from build123d import *

# Parameters (mm, degrees)
BOSS_EXTRUDE1_DEPTH   = 3
CUT_EXTRUDE1_REACH    = 84.517
SKETCH2_R             = 1
SKETCH2_R_2           = 1.25
SKETCH3_R             = 10
BOSS_EXTRUDE2_DEPTH   = 15
BODY_MOVE_COPY2_ANGLE = 90


with BuildPart() as part:
    # Sketch1 → Boss-Extrude1 (new body)
    with BuildSketch(Plane(origin=(0, 0, 0), x_dir=(1, 0, 0), z_dir=(0, 1, 0))):
        with BuildLine():
            Line((60, -20), (0, -20))
            ThreePointArc((0, -20), (-20, 0), (0, 20))
            Line((0, 20), (60, 20))
            Line((60, 20), (80, 0))
            Line((80, 0), (60, -20))
        make_face()
    extrude(amount=BOSS_EXTRUDE1_DEPTH)

    # Sketch2 → Cut-Extrude1 (cut, up to next)
    with BuildSketch(Plane(origin=(0, 3, 0), x_dir=(1, 0, 0), z_dir=(0, 1, 0)), mode=Mode.PRIVATE) as cut_extrude1_sk1:
        with Locations(Location((0, 0, 0), (0, 0, 270))):
            Circle(SKETCH2_R)
    cut_extrude1_tool1 = extrude(cut_extrude1_sk1.sketch, amount=-CUT_EXTRUDE1_REACH, mode=Mode.PRIVATE) & part.part
    # Sketch2 → Cut-Extrude1 (cut, up to next)
    with BuildSketch(Plane(origin=(0, 3, 0), x_dir=(1, 0, 0), z_dir=(0, 1, 0)), mode=Mode.PRIVATE) as cut_extrude1_sk2:
        with Locations(Location((0, 7, 0), (0, 0, 270))):
            Circle(SKETCH2_R_2)
    cut_extrude1_tool2 = extrude(cut_extrude1_sk2.sketch, amount=-CUT_EXTRUDE1_REACH, mode=Mode.PRIVATE) & part.part
    # Sketch2 → Cut-Extrude1 (cut, up to next)
    with BuildSketch(Plane(origin=(0, 3, 0), x_dir=(1, 0, 0), z_dir=(0, 1, 0)), mode=Mode.PRIVATE) as cut_extrude1_sk3:
        with Locations(Location((7.001, 0.001, 0), (0, 0, 270))):
            Circle(SKETCH2_R_2)
    cut_extrude1_tool3 = extrude(cut_extrude1_sk3.sketch, amount=-CUT_EXTRUDE1_REACH, mode=Mode.PRIVATE) & part.part
    # Sketch2 → Cut-Extrude1 (cut, up to next)
    with BuildSketch(Plane(origin=(0, 3, 0), x_dir=(1, 0, 0), z_dir=(0, 1, 0)), mode=Mode.PRIVATE) as cut_extrude1_sk4:
        with Locations(Location((0.002, -7, 0), (0, 0, 270))):
            Circle(SKETCH2_R_2)
    cut_extrude1_tool4 = extrude(cut_extrude1_sk4.sketch, amount=-CUT_EXTRUDE1_REACH, mode=Mode.PRIVATE) & part.part
    # Sketch2 → Cut-Extrude1 (cut, up to next)
    with BuildSketch(Plane(origin=(0, 3, 0), x_dir=(1, 0, 0), z_dir=(0, 1, 0)), mode=Mode.PRIVATE) as cut_extrude1_sk5:
        with Locations(Location((-6.999, -0.001, 0), (0, 0, 270))):
            Circle(SKETCH2_R_2)
    cut_extrude1_tool5 = extrude(cut_extrude1_sk5.sketch, amount=-CUT_EXTRUDE1_REACH, mode=Mode.PRIVATE) & part.part
    add(cut_extrude1_tool1.solids().sort_by_distance((0, 3, 0))[0], mode=Mode.SUBTRACT)
    add(cut_extrude1_tool2.solids().sort_by_distance((0, 3, -7))[0], mode=Mode.SUBTRACT)
    add(cut_extrude1_tool3.solids().sort_by_distance((7.001, 3, -0.001))[0], mode=Mode.SUBTRACT)
    add(cut_extrude1_tool4.solids().sort_by_distance((0.002, 3, 7))[0], mode=Mode.SUBTRACT)
    add(cut_extrude1_tool5.solids().sort_by_distance((-6.999, 3, 0.001))[0], mode=Mode.SUBTRACT)

    # Sketch3 → Boss-Extrude2 (add)
    with BuildSketch(Plane.XZ):
        with Locations(Location((0, 0, 0), (0, 0, 90))):
            Circle(SKETCH3_R)
    extrude(amount=BOSS_EXTRUDE2_DEPTH)


with BuildPart() as part_1:
    # Body-Move/Copy2: moved
    add(part.part.rotate(Axis((0, 0, 0), (1, 0, 0)), BODY_MOVE_COPY2_ANGLE))


with BuildPart() as part_2:
    # Body-Move/Copy3: moved
    add(part_1.part.moved(Location((0, 0, -3))))


solid = part_2.part
Source: CAD feature listing. Evaluate the final solid. Frame: model axes, mm. A direction names the side the tool comes from. Coordinates: 2 decimals unless noted, no trailing zeros. Loops run counter-clockwise (first coordinate to the right, second up) from the corner with the lowest first, then second, coordinate; pieces in that order, holes last. Notation, with made-up numbers: (-35, 27.5) -> (-19, 27.5) arc R7 cw to (-19, 40.5) -> close; hole circle Ø3 at (88.5, -7). An arc over 180 degrees is marked (long way). Answer in a Markdown table with one row per item. Add a question column.
Q1. Contact query for flat-ended pins moving along their axis: pin 1 Ø1.2 at (x, y) = (0, -7) entering from +Z; pin 2 Ø2 at (x, y) = (55, 4.5) entering from -Z; pin 3 Ø2 at (x, y) = (7, 0.5) entering from +Z; pin 4 Ø6 at (y, z) = (-7, -13.5) entering from +X. Output: stop coordinate, or through.
Q2. Section C-C on x = 20.5. Return the cut outline in (y, z).
Q3. Reachability of faces 5 (the face through (0.05, 8.25, -1.48)), 6 (the face through (9.76, 2.17, -10.4)), 7 (the face through (31, 0, 0)) from +Z, -Z, +X, -X, +Y, -Y: full face, straight path, thin tool, end or side. Return the list, or none.
Q4. Section D-D on y = -13. Return the cut outline in (x, z).
Q5. Section A-A on y = 7. Return the cut outline in (x, z) (3 decimals), and give its area (3 significant figures).
Q6. Ray query, line 1 along X through (y, z) = (0, -0.95); line 2 along Z through (x, y) = (25, -6.5); line 3 along X through (y, z) = (0, -11.75). Return the intervals inside material, ascending.
Q7. Pull-direction query (X, two-part tool) for faces 1 (the face through (-20, 0, -2)), 2 (the face through (30, -20, -2)), 3 (the face through (70, -10, -2)), 4 (the face through (0, 0, -3)); classes: pulls with the +X half, pulls with the -X half, needs draft (parallel to the pull), parting line crosses it, or undercut.
Q8. Section B-B on z = -7. Return the cut outline in (x, y).
Computed values:
| question | item | result |
|---|---|---|
| 1 | pin 1 | stops at z = -3 |
| 1 | pin 2 | stops at z = -3 |
| 1 | pin 3 | stops at z = 0 |
| 1 | pin 4 | stops at x = 9.17 |
| 2 | outline | (-20, -3) -> (20, -3) -> (20, 0) -> (-20, 0) -> close |
| 3 | face 5 | +Z |
| 3 | face 6 | -Z |
| 3 | face 7 | +Z, +X, -X, +Y, -Y |
| 4 | outline | (-15.2, -3) -> (67, -3) -> (67, 0) -> (-15.2, 0) -> close |
| 5 | outline | (-18.735, -3) -> (-7.141, -3) -> (-7.141, -18) -> (7.141, -18) -> (7.141, -3) -> (73, -3) -> (73, 0) -> (1.25, 0) -> (1.25, -3) -> (-1.25, -3) -> (-1.25, 0) -> (-18.735, 0) -> close |
| 5 | area | 482 mm^2 |
| 6 | line 1 | x = -20 to -8.25, -5.75 to -1, 1 to 5.75, 8.25 to 80 |
| 6 | line 2 | z = -3 to 0 |
| 6 | line 3 | x = -10 to 10 |
| 7 | face 1 | pulls with the -X half |
| 7 | face 2 | needs draft |
| 7 | face 3 | pulls with the +X half |
| 7 | face 4 | undercut |
| 8 | outline | circle Ø20 at (0, 0) |
